Check sheet for the modelled part. Datum: model origin and axes. Units: mm. A direction names the side the tool comes from. Coordinates: 2 decimals unless noted, no trailing zeros. Order: outer loops, then holes, each group sorted by start corner. A loop starts at its lowest first (then second) coordinate and runs counter-clockwise, first axis right, second up.
Autodesk Fusion 360 part; units mm, degrees
sketch "Sketch1" plane through (0, 0, 0) normal (1, 0, 0) x (0, 1, 0)
  line L0 (0, 0) -> (0, 14.3282)
  line L1 (0, 14.3282) -> (103.0489, 14.3282)
  line L2 (103.0489, 14.3282) -> (103.0489, 0)
  line L3 (51.5244, 0) -> (51.5244, 7.1641) construction
  line L4 (51.5244, 7.1641) -> (72.6846, 7.1641)
  line L5 (72.6846, 7.1641) -> (80.2757, 0)
  line L6 (51.5244, 7.1641) -> (30.3643, 7.1641)
  line L7 (30.3643, 7.1641) -> (22.7732, 0)
  line L8 (103.0489, 0) -> (80.2757, 0)
  line L9 (22.7732, 0) -> (0, 0)
extrude "Extrude1" add sketch "Sketch1" along normal blind 80
sketch "Sketch2" plane through (0, 0, 14.3282) normal (0, 0, 1) x (-1, 0, 0)
  circle A0 centre (-13.5834, -13.8842) radius 5.0923
extrude "Extrude2" cut sketch "Sketch2" against normal through all
pattern_linear "R-Pattern1" count 3 spacing 39.4785 along (0, 1, 0) count 2 spacing 45.613 along (1, 0, 0) of "Extrude2"
(1) Release check for a two-part mould opening along X. For faces 1 (the flat face through (0, 51, 9)), 2 (the flat face through (39, 103.049, 7)), 3 (the flat face through (80, 51, 9)), 4 (the cylindrical face through (14.246, 87.792, 7.264)) record: +X half, -X half, draft (parallel to the pull), parting line (faces both ways), or undercut.
Filled in:
face 1: -X half
face 2: draft
face 3: +X half
face 4: undercut
(2) Cross-section at B-B (y = 90.5). Enter the section's corners in (x, z), and give its area (3 significant figures).
Filled in:
outline: (0, 0) - (9.06, 0) - (9.06, 14.33) - (0, 14.33) - close; (18.11, 0) - (54.67, 0) - (54.67, 14.33) - (18.11, 14.33) - close; (63.72, 0) - (80, 0) - (80, 14.33) - (63.72, 14.33) - close
area: 887 mm2
(3) Thickness scan on probe 1 along Y at (x, z) = (60.5, 13); probe 2 along Y at (x, z) = (63, 8.75); probe 3 along Z at (x, y) = (71.5, 66). Record the ranges inside material, lowest first.
Filled in:
probe 1: y = 0 to 8.96, 18.81 to 48.44, 58.29 to 87.92, 97.76 to 103.05
probe 2: y = 0 to 10.5, 17.27 to 49.98, 56.75 to 89.46, 96.23 to 103.05
probe 3: z = 7.16 to 14.33
(4) Go/stop test with a flat-tipped pin: P1, Ø12.5, axis at x = 42.5, y = 52, coming from the -Z side. Record where the tip stops, or that it passes through.
Filled in:
P1: stops at z = 7.16
(5) Cross-section at D-D (x = 14). Enter the section's corners in (y, z).
Filled in:
outline: (0, 0) - (8.81, 0) - (8.81, 14.33) - (0, 14.33) - close; (18.96, 0) - (22.77, 0) - (30.36, 7.16) - (48.29, 7.16) - (48.29, 14.33) - (18.96, 14.33) - close; (58.44, 7.16) - (72.68, 7.16) - (80.28, 0) - (87.77, 0) - (87.77, 14.33) - (58.44, 14.33) - close; (97.92, 0) - (103.05, 0) - (103.05, 14.33) - (97.92, 14.33) - close
(6) Cross-section at C-C (x = 33.5). Enter the section's corners in (y, z), and give its area (3 significant figures).
Filled in:
outline: (0, 0) - (22.77, 0) - (30.36, 7.16) - (72.68, 7.16) - (80.28, 0) - (103.05, 0) - (103.05, 14.33) - (0, 14.33) - close
area: 1,120 mm2
(7) Cross-section at A-A (z = 1.25). Enter the section's corners in (x, y), and give its area (3 significant figures).
Filled in:
outline: (0, 0) - (80, 0) - (80, 24.1) - (0, 24.1) - close; (0, 78.95) - (80, 78.95) - (80, 103.05) - (0, 103.05) - close; hole circle Ø10.18 at (13.58, 13.88); hole circle Ø10.18 at (13.58, 92.84); hole circle Ø10.18 at (59.2, 13.88); hole circle Ø10.18 at (59.2, 92.84)
area: 3,530 mm2
(8) Tool access check on faces 5 (the cylindrical face through (18.67, 13.66, 7.26)), 6 (the flat face through (39.44, 26.62, 3.63)). Record the directions out of +Z, -Z, +X, -X, +Y, -Y that give a thin tool (end or side, any length) a straight path to the whole face; none if there is none.
Filled in:
face 5: +Z, -Z
face 6: -Z, +X, -X
